CAD build for the part. Positions are in the model's coordinates, mm. Face numbers are marked on the shaded views. A direction names the side the tool comes from. Give positions to 0.01 mm unless a question says otherwise; leave off trailing zeros. Loops run counter-clockwise (first coordinate to the right, second up) from the corner with the lowest first, then second, coordinate; pieces in that order, holes last. Notation, with made-up numbers: (-28, 67) -> (11, 67) arc R30 ccw to (11, 101) -> close; hole circle Ø10 at (21.25, -2). An arc over 180 degrees is marked (long way). Use one line per item in the form item = value.
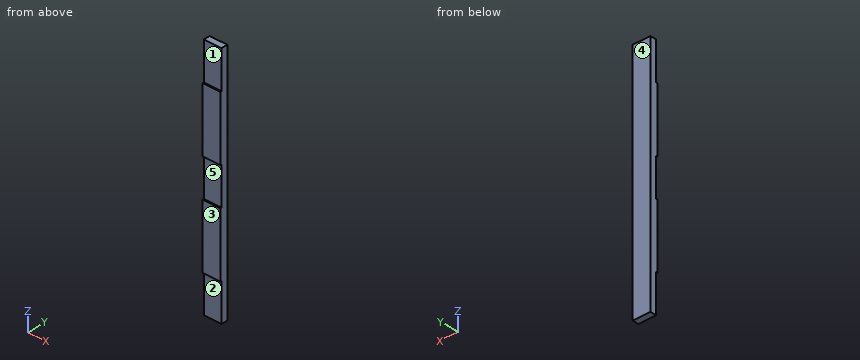
```python
from build123d import *

# Parameters (mm, degrees)
F0_W     = 88.9
F0_H     = 1219.2
F1_DEPTH = 19.05
F2_W     = 88.9
F2_H     = 190.5
F3_DEPTH = 6.35


with BuildPart() as f1:
    # F0 (on Front) → F1 (new body, symmetric)
    with BuildSketch(Plane.XZ):
        Rectangle(F0_W, F0_H)
    extrude(amount=F1_DEPTH, both=True)

    # F2 (on face) → F3 (cut)
    with BuildSketch(Plane.XZ.offset(19.05)):
        with Locations((0, -514.35)):
            Rectangle(F2_W, F2_H)
        Rectangle(F2_W, F2_H)
        with Locations((0, 514.35)):
            Rectangle(F2_W, F2_H)
    extrude(amount=-F3_DEPTH, mode=Mode.SUBTRACT)


solid = f1.part
```
1. Drill centre lines: line 1 (Z direction, x = -11.5, y = -14); line 2 (Y direction, x = -2.5, z = -85). Where is each one in solid material? Low to high.
Result sheet:
line_1 = -419.1 to -95.25, 95.25 to 419.1
line_2 = -12.7 to 19.05
2. Tool access for the marked faces 1, 2 and 3: list every direction of +Z, -Z, +X, -X, +Y, -Y with a clear straight run to the whole face (end or side of a thin tool).
Result sheet:
face_1 = +Z, +X, -X, -Y
face_2 = -Z, +X, -X, -Y
face_3 = +Z, -Z, +X, -X, -Y
3. Cut at A-A, the plane x = -19.5. Write the cut outline in (y, z), then the cut area to 3 significant figures.
Result sheet:
outline = (-19.05, -419.1) -> (-12.7, -419.1) -> (-12.7, -609.6) -> (19.05, -609.6) -> (19.05, 609.6) -> (-12.7, 609.6) -> (-12.7, 419.1) -> (-19.05, 419.1) -> (-19.05, 95.25) -> (-12.7, 95.25) -> (-12.7, -95.25) -> (-19.05, -95.25) -> close
area = 42,800 mm^2
4. Drop flat-ended pins along their axis: P1, Ø7, axis at x = 11, y = -17, coming from the -Z side; P2, Ø4, axis at x = -7, z = -468, coming from the -Y side; P3, Ø1.9, axis at x = 2.5, y = -15.5, coming from the +Z side. Give the stop position or say it passes through.
Result sheet:
P1 = -419.1
P2 = -12.7
P3 = 419.1
5. Cut at B-B, the plane z = 23. Write the cut outline in (x, y), then the cut area to 3 significant figures.
Result sheet:
outline = (-44.45, -12.7) -> (44.45, -12.7) -> (44.45, 19.05) -> (-44.45, 19.05) -> close
area = 2,820 mm^2
6. Mould opens along Z. For the marked faces 4 and 5 say: pulls with the +Z half, pulls with the -Z half, needs draft (parallel to the pull), parting line crosses it, or undercut.
Result sheet:
face_4 = needs draft
face_5 = undercut
